Geometry: final body of the model. Coordinates: model frame, mm. Face numbers are marked on the shaded views. A direction names the side the tool comes from. Give positions to 0.01 mm unless a question says otherwise; leave off trailing zeros. Loops run counter-clockwise (first coordinate to the right, second up) from the corner with the lowest first, then second, coordinate; pieces in that order, holes last.
1. Draft query along Z for the marked faces 1, 2 and 3. Return one class per face: +Z half, -Z half, draft (parallel to the pull), parting line (faces both ways), or undercut.
2. Access query for the marked faces 4 and 5. Directions: +Z, -Z, +X, -X, +Y, -Y. A direction counts if a zero-diameter tool reaches every point of the face in a straight line with its end or side. Return the directions, or none.
3. First-contact query: P1, Ø1, axis at y = 1.5, z = 12, coming from the -X side; P2, Ø3, axis at x = 5, z = 14, coming from the +Y side; P3, Ø10, axis at y = 16.5, z = 33.5, coming from the -X side. Flat tips, straight axial feed; report the tip coordinate or a pass-through.
4. Section D-D, the plane y = 25.5. Output: boundary loops of the cut face in (x, z), then the cut area to 3 significant figures.
5. Section B-B, the plane x = -13. Output: boundary loops of the cut face in (y, z), then the cut area to 3 significant figures.
6. Section C-C, the plane z = 34. Output: boundary loops of the cut face in (x, y), then the cut area to 3 significant figures.
7. Material intervals for line 1 along Z through (x, y) = (1, 22.5); line 2 along X through (y, z) = (29, 26.5); line 3 along Z through (x, y) = (10.5, 34.5), sorted ascending.
8. Section A-A, the plane y = 6. Output: boundary loops of the cut face in (x, z), then the cut area to 3 significant figures.
from build123d import *

# Parameters (mm, degrees)
EXTRUDE001_DEPTH = 4
EXTRUDE002_DEPTH = 4
EXTRUDE003_DEPTH = 44.5
EXTRUDE_DEPTH    = 36.5
CHAMFER_SIZE     = 3
CHAMFER001_SIZE  = 3
CHAMFER002_SIZE  = 3
CHAMFER003_SIZE  = 3


with BuildPart() as extrude001:
    # Sketch001 (on Face14 of Extrude) → Extrude001 (new body)
    with BuildSketch(Plane.XY.offset(36.5)):
        Polygon((-33, 36), (33, 36), (33, 24), (27.166667, -4), (-27.166667, -4), (-33, 24), align=None)
    extrude(amount=EXTRUDE001_DEPTH)


with BuildPart() as extrude002:
    # Sketch002 (on Face13 of Extrude) → Extrude002 (new body)
    with BuildSketch(Plane(origin=(0, 0, 0), x_dir=(1, 0, 0), z_dir=(0, 0, -1))):
        Polygon((-33, -36), (-33, -24), (-27.166667, 4), (27.166667, 4), (33, -24), (33, -36), align=None)
    extrude(amount=EXTRUDE002_DEPTH)


with BuildPart() as extrude003:
    # Sketch003 (on Face8 of Extrude002) → Extrude003 (new body)
    with BuildSketch(Plane(origin=(0, 0, -4), x_dir=(1, 0, 0), z_dir=(0, 0, -1))):
        with BuildLine():
            Line((27.166667, 4), (47, 4))
            Line((47, -36), (47, 4))
            Line((44, -36), (47, -36))
            ThreePointArc((44, -36), (39, -31), (34, -36))
            Line((33, -36), (34, -36))
            Line((33, -24), (33, -36))
            Line((27.166667, 4), (33, -24))
        make_face()
    extrude(amount=-EXTRUDE003_DEPTH)


with BuildPart() as chamfer003:
    # Sketch → Extrude (new body)
    with BuildSketch(Plane.XY):
        Polygon((-24, 0), (24, 0), (29, 24), (29, 36), (33, 36), (33, 24), (27.166667, -4), (-27.166667, -4), (-33, 24), (-33, 36), (-29, 36), (-29, 24), align=None)
    extrude(amount=EXTRUDE_DEPTH)

    # Fusion: union Extrude001, Extrude002, Extrude003
    add(extrude001.part)
    add(extrude002.part)
    add(extrude003.part)

    # Chamfer
    chamfer_edges = [chamfer003.edges().sort_by_distance(p)[0] for p in [
        (0, 36, 36.5),
    ]]
    chamfer(chamfer_edges, length=CHAMFER_SIZE)

    # Chamfer001
    chamfer001_edges = [chamfer003.edges().sort_by_distance(p)[0] for p in [
        (0, 36, 0),
    ]]
    chamfer(chamfer001_edges, length=CHAMFER001_SIZE)

    # Chamfer002
    chamfer002_edges = [chamfer003.edges().sort_by_distance(p)[0] for p in [
        (29, 36, 38),
        (29, 36, 18.25),
        (29, 36, -1.5),
    ]]
    chamfer(chamfer002_edges, length=CHAMFER002_SIZE)

    # Chamfer003
    chamfer003_edges = [chamfer003.edges().sort_by_distance(p)[0] for p in [
        (-29, 36, 38),
        (-29, 36, 18.25),
        (-29, 36, -1.5),
    ]]
    chamfer(chamfer003_edges, length=CHAMFER003_SIZE)


solid = chamfer003.part
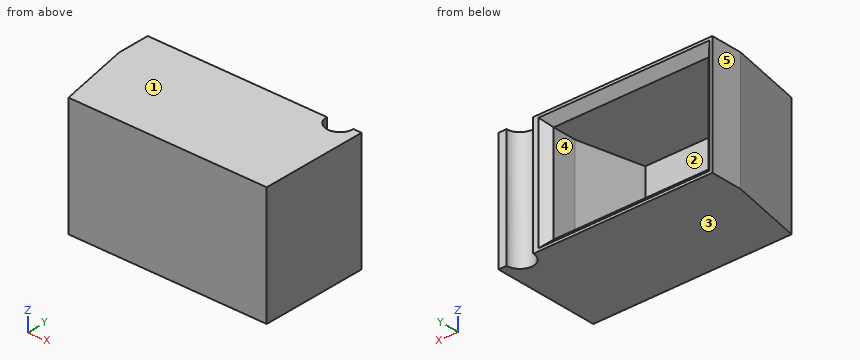
Answers below:
1. face 1: +Z half
1. face 2: undercut
1. face 3: -Z half
2. face 4: +Y
2. face 5: +Z, -Z, -X, +Y, -Y
3. P1: stops at x = -28.42
3. P2: stops at y = 0
3. P3: stops at x = -32.48
4. outline: (-33, -4) - (47, -4) - (47, 40.5) - (-33, 40.5) - close; hole (-29, 0) - (29, 0) - (29, 36.5) - (-29, 36.5) - close
4. area: 1,440 mm2
5. outline: (-4, -4) - (36, -4) - (36, -3) - (33, 0) - (0, 0) - (0, 36.5) - (33, 36.5) - (36, 39.5) - (36, 40.5) - (-4, 40.5) - close
5. area: 457 mm2
6. outline: (-33, 24) - (-27.17, -4) - (47, -4) - (47, 36) - (44, 36) arc R5 cw to (34, 36) - (32, 36) - (29, 33) - (29, 24) - (24, 0) - (-24, 0) - (-29, 24) - (-29, 33) - (-32, 36) - (-33, 36) - close
6. area: 1,100 mm2
7. line 1: z = -4 to 0, 36.5 to 40.5
7. line 2: x = -33 to -29, 29 to 47
7. line 3: z = -4 to -1.5, 38 to 40.5
8. outline: (-29.25, -4) - (47, -4) - (47, 40.5) - (-29.25, 40.5) - close; hole (-25.25, 0) - (25.25, 0) - (25.25, 36.5) - (-25.25, 36.5) - close
8. area: 1,550 mm2
